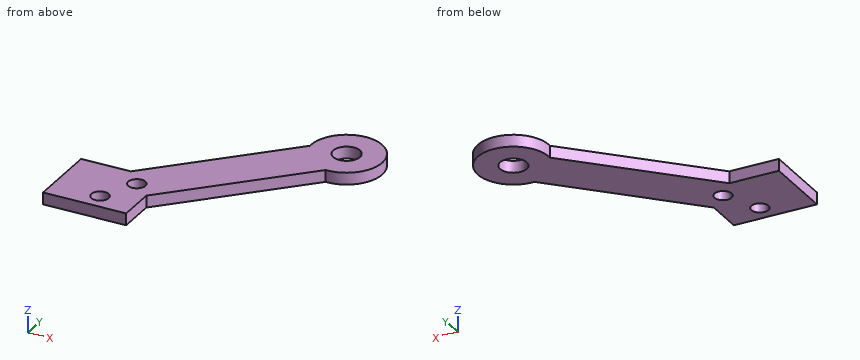
```python
from build123d import *

# Parameters (mm, degrees)
SKETCH1_R                         = 6
SKETCH1_R_2                       = 2.25
FOLLOWER_SEAT_D4P5_DEPTH          = 2
CARRIAGE_TO_FOLLOWER_BRIDGE_DEPTH = 2
SKETCH3_W                         = 14
SKETCH3_H                         = 12
CARRIAGE_ATTACHMENT_PAD_DEPTH     = 2
SKETCH5_R                         = 1.45
STOP_MOUNT_D2P9_THROUGH_DEPTH     = 2.01


with BuildPart() as part:
    # Sketch1 → Follower_Seat_D4p5 (new body)
    with BuildSketch(Plane.XY):
        with Locations((50, 50)):
            Circle(SKETCH1_R)
        with Locations((50, 50)):
            Circle(SKETCH1_R_2, mode=Mode.SUBTRACT)
    extrude(amount=FOLLOWER_SEAT_D4P5_DEPTH)

    # Sketch2 → Carriage_To_Follower_Bridge (add)
    with BuildSketch(Plane.XY):
        Polygon((21.171572875, 26.828427125), (44.171572875, 49.828427125), (49.828427125, 44.171572875), (26.828427125, 21.171572875), align=None)
    extrude(amount=CARRIAGE_TO_FOLLOWER_BRIDGE_DEPTH)

    # Sketch3 → Carriage_Attachment_Pad (add)
    with BuildSketch(Plane.XY):
        with Locations((23, 24)):
            Rectangle(SKETCH3_W, SKETCH3_H)
    extrude(amount=CARRIAGE_ATTACHMENT_PAD_DEPTH)

    # Sketch5 → Stop_Mount_D2p9_Through (cut)
    with BuildSketch(Plane.XY.offset(2)):
        with Locations((24, 21)):
            Circle(SKETCH5_R)
        with Locations((27, 27)):
            Circle(SKETCH5_R)
    extrude(amount=-STOP_MOUNT_D2P9_THROUGH_DEPTH, mode=Mode.SUBTRACT)


solid = part.part
```
Source: CAD feature listing. Evaluate the final solid. Frame: model axes, mm. Coordinates: 2 decimals unless noted, no trailing zeros. Loops run counter-clockwise (first coordinate to the right, second up) from the corner with the lowest first, then second, coordinate; pieces in that order, holes last. Notation, with made-up numbers: M -15.75,71 L 28.25,71 A23 ccw 28.25,96 Z; hole C 2,10.5 d5. An arc over 180 degrees is marked long. Use CSV: the item, a comma, the result in double quotes.
(1) Line query: line 1 (Y direction, x = 50, z = 1.65); line 2 (Y direction, x = 24, z = 1.4); line 3 (Y direction, x = 22, z = 0.15). Output: solid intervals per line, ascending. Write a range as [from, to].
Answers follow:
line 1,"[44, 47.75], [52.25, 56]"
line 2,"[18, 19.55], [22.45, 30]"
line 3,"[18, 30]"
(2) Cut plane C-C on y = 27. Return loops of the section in (x, z).
Answers follow:
outline,"M 16,0 L 25.55,0 L 25.55,2 L 16,2 Z; M 28.45,0 L 32.66,0 L 32.66,2 L 28.45,2 Z"
(3) Cut plane D-D on x = 36. Return loops of the section in (y, z).
Answers follow:
outline,"M 30.34,0 L 41.66,0 L 41.66,2 L 30.34,2 Z"
(4) Cut plane A-A on y = 21. Return loops of the section in (x, z), and give its area (3 significant figures).
Answers follow:
outline,"M 16,0 L 22.55,0 L 22.55,2 L 16,2 Z; M 25.45,0 L 30,0 L 30,2 L 25.45,2 Z"
area,"22.2 mm²"
(5) Cut plane B-B on z = 0.65. Return loops of the section in (x, y), and give its area (3 significant figures).
Answers follow:
outline,"M 16,18 L 30,18 L 30,24.34 L 49.67,44.01 A6 ccw long 44.01,49.67 L 24.34,30 L 16,30 Z; hole C 24,21 d2.9; hole C 27,27 d2.9; hole C 50,50 d4.5"
area,"450 mm²"
(6) Contact query for flat-ended pins moving along their axis: pin 1 (4.5 mm diameter, centred on x = 24, y = 21, fed in from +Z); pin 2 (1.7 mm diameter, centred on x = 27, y = 27, fed in from +Z). Output: stop coordinate, or through.
Answers follow:
pin 1,"z = 2"
pin 2,"through"
